Geometry: final body of the model. Coordinates: model frame, mm. A direction names the side the tool comes from. Round coordinates to 2 decimals unless told otherwise and drop trailing zeros. Loops run counter-clockwise (first coordinate to the right, second up) from the corner with the lowest first, then second, coordinate; pieces in that order, holes last. Notation, with made-up numbers: (18, -27) -> (26, -27) arc R28 ccw to (26, -6) -> close; hole circle Ø1 at (42, 74). An arc over 180 degrees is marked (long way). Answer in a Markdown table with one row per item.
```python
from build123d import *

# Parameters (mm, degrees)
SKETCH2_W           = 40.64
SKETCH2_H           = 40.64
BOSS_EXTRUDE1_DEPTH = 38.1
SKETCH3_W           = 40.64
SKETCH3_H           = 40.64
SKETCH3_W_2         = 39.116
SKETCH3_H_2         = 39.116
CUT_EXTRUDE1_DEPTH  = 35.56
SKETCH4_R           = 19.177
CUT_EXTRUDE3_DEPTH  = 35.56


with BuildPart() as part:
    # Sketch2 → Boss-Extrude1 (new body)
    with BuildSketch(Plane.XY):
        with Locations((0.436989247, 1.966451613)):
            Rectangle(SKETCH2_W, SKETCH2_H)
    extrude(amount=BOSS_EXTRUDE1_DEPTH)

    # Sketch3 → Cut-Extrude1 (cut)
    with BuildSketch(Plane.XY.offset(38.1)):
        with Locations((0.436989247, 1.966451613)):
            Rectangle(SKETCH3_W, SKETCH3_H)
        with Locations((0.466860662, 2.084424142)):
            Rectangle(SKETCH3_W_2, SKETCH3_H_2, mode=Mode.SUBTRACT)
    extrude(amount=-CUT_EXTRUDE1_DEPTH, mode=Mode.SUBTRACT)

    # Sketch4 → Cut-Extrude3 (cut)
    with BuildSketch(Plane.XY.offset(38.1)):
        with Locations((0.37530299, 1.719706585)):
            Circle(SKETCH4_R)
    extrude(amount=-CUT_EXTRUDE3_DEPTH, mode=Mode.SUBTRACT)


solid = part.part
```
Item 1: Section query C-C, the plane y = -1.5. Output: boundary loops of the cut face in (x, z), and give its area (3 significant figures).
Ans:
| item | result |
|---|---|
| outline | (-19.88, 0) -> (20.76, 0) -> (20.76, 2.54) -> (20.02, 2.54) -> (20.02, 38.1) -> (19.28, 38.1) -> (19.28, 2.54) -> (-18.53, 2.54) -> (-18.53, 38.1) -> (-19.09, 38.1) -> (-19.09, 2.54) -> (-19.88, 2.54) -> close |
| area | 150 mm2 |
Item 2: Set-up query: faces 4 (the flat face through (20.025, 2, 21)), 5 (the flat face through (0, 2, 2.54)), 6 (the flat face through (0, 21.642, 21)), 7 (the flat face through (-19.091, 2, 21)), 8 (the flat face through (-4, -17.474, 21)). Return all of +Z, -Z, +X, -X, +Y, -Y with unobstructed straight access to the full face (end or side cutting, diameter ignored); none if empty.
Ans:
| item | result |
|---|---|
| face 4 | +Z, +X, +Y, -Y |
| face 5 | +Z |
| face 6 | +Z, +X, -X, +Y |
| face 7 | +Z, -X, +Y, -Y |
| face 8 | +Z, +X, -X, -Y |
Item 3: Section query B-B, the plane x = 6.5. Output: boundary loops of the cut face in (y, z).
Ans:
| item | result |
|---|---|
| outline | (-18.35, 0) -> (22.29, 0) -> (22.29, 2.54) -> (21.64, 2.54) -> (21.64, 38.1) -> (19.89, 38.1) -> (19.89, 2.54) -> (-16.45, 2.54) -> (-16.45, 38.1) -> (-17.47, 38.1) -> (-17.47, 2.54) -> (-18.35, 2.54) -> close |
Item 4: Mould query, pull axis X, two halves, no side actions, for faces 1 (the flat face through (20.757, 2, 1)), 2 (the cylindrical face through (-3.78, -17, 20.57)), 3 (the flat face through (2, 21, 38.1)). Classes: released by +X, released by -X, zero draft, split by the parting line, or undercut.
Ans:
| item | result |
|---|---|
| face 1 | released by +X |
| face 2 | undercut |
| face 3 | zero draft |
Item 5: First-contact query: P1, Ø10, axis at x = -0.5, z = 33, coming from the -Y side; P2, Ø12, axis at y = -9.5, z = 22.5, coming from the +X side; P3, Ø2, axis at y = 8, z = 32, coming from the -X side. Flat tips, straight axial feed; report the tip coordinate or a pass-through.
Ans:
| item | result |
|---|---|
| P1 | y = -17.47 |
| P2 | x = 20.02 |
| P3 | x = -19.09 |
Item 6: Ray query, L1, parallel to X at y = 1.5, z = 25.5; L2, parallel to Z at x = 1.5, y = 16.5; L3, parallel to X at y = 9.5, z = 21. Return the intervals inside material, ascending.
Ans:
| item | result |
|---|---|
| L1 | -19.09 to -18.8, 19.55 to 20.02 |
| L2 | 0 to 2.54 |
| L3 | -19.09 to -17.15, 17.9 to 20.02 |
Item 7: Section query A-A, the plane z = 16. Output: boundary loops of the cut face in (x, y).
Ans:
| item | result |
|---|---|
| outline | (-19.09, -17.47) -> (20.02, -17.47) -> (20.02, 21.64) -> (-19.09, 21.64) -> close; hole circle Ø38.35 at (0.38, 1.72) |
